from build123d import *

# Parameters (mm, degrees)
F0_W     = 71.2
F0_H     = 88
F1_DEPTH = 1.5
F2_W     = 71.2
F2_H     = 88
F2_W_2   = 67.2
F2_H_2   = 84
F3_DEPTH = 4


with BuildPart() as f1:
    # F0 (on Top) → F1 (new body)
    with BuildSketch(Plane.XY):
        with BuildLine():
            Line((35.4853983939, 37.8176547885), (-32.7146016061, 37.8176547885))
            ThreePointArc((-32.7146016061, 37.8176547885), (-35.5430287309, 36.6460819132), (-36.7146016061, 33.8176547885))
            Line((-36.7146016061, 33.8176547885), (-36.7146016061, -51.1823452115))
            ThreePointArc((-36.7146016061, -51.1823452115), (-35.5430287309, -54.0107723363), (-32.7146016061, -55.1823452115))
            Line((-32.7146016061, -55.1823452115), (35.4853983939, -55.1823452115))
            ThreePointArc((35.4853983939, -55.1823452115), (38.3138255186, -54.0107723363), (39.4853983939, -51.1823452115))
            Line((39.4853983939, -51.1823452115), (39.4853983939, 33.8176547885))
            ThreePointArc((39.4853983939, 33.8176547885), (38.3138255186, 36.6460819132), (35.4853983939, 37.8176547885))
        make_face()
        with Locations((1.3853983939, -8.6823452115)):
            Rectangle(F0_W, F0_H, mode=Mode.SUBTRACT)
        with Locations((1.3853983939, -8.6823452115)):
            Rectangle(F0_W, F0_H)
    extrude(amount=F1_DEPTH)

    # F2 (on face) → F3 (join)
    with BuildSketch(Plane.XY.offset(1.5)):
        with Locations((1.3853983939, -8.6823452115)):
            Rectangle(F2_W, F2_H)
        with Locations((1.3853983939, -8.6823452115)):
            Rectangle(F2_W_2, F2_H_2, mode=Mode.SUBTRACT)
    extrude(amount=F3_DEPTH)


solid = f1.part
The listing builds one solid part. Answer for the finished solid, in the listing's coordinates (mm). A direction names the side the tool comes from. Coordinates: 2 decimals unless noted, no trailing zeros. Order: outer loops, then holes, each group sorted by start corner. A loop starts at its lowest first (then second) coordinate and runs counter-clockwise, first axis right, second up. Notation, with made-up numbers: (34, 45.25) -> (49, 45.25) arc R33 ccw to (49, 77.25) -> close; hole circle Ø8 at (54, -11). An arc over 180 degrees is marked (long way). Answer in a Markdown table with one row per item. Add a question column.
Item 1: Which of the six approach directions +Z, -Z, +X, -X, +Y, -Y give full straight-line access (tool end or side, diameter ignored) to faces 5 (the face through (1, -8, 0)), 6 (the face through (-35.574, -53.98, 0.74)), 7 (the face through (1, -8, 1.5)), 8 (the face through (1, 35.318, 3)), 9 (the face through (-34.215, -9, 3))?
Item 2: Find section C-C (y = -13.5). Write down the section's boundary in (x, z), then the cut area to 3 significant figures.
Item 3: Find section B-B (x = 30.5). Write down the section's boundary in (y, z).
Item 4: Find section A-A (z = 2.35). Write down the section's boundary in (x, y), then the cut area to 3 significant figures.
Item 5: Each of these flat-tipped pins is pushed along its axis until it touches: P1, Ø2, axis at y = -11.5, z = 3.5, coming from the +X side; P2, Ø23, axis at x = 15.5, y = -22.5, coming from the +Z side; P3, Ø1.2, axis at x = 14, z = 4.5, coming from the -Y side. Where does it stop, or does it pass through?
Item 6: Determine the mould class of faces 1 (the face through (36.985, -9, 3)), 2 (the face through (1, -50.682, 3)), 3 (the face through (-35.51, 36.68, 0.74)), 4 (the face through (1, -52.682, 3)) for opening direction Y: +Y half, -Y half, draft (parallel to the pull), parting line (faces both ways), or undercut.
Item 7: Find the intervals of material crossed by L1, parallel to X at y = -42.5, z = 2.2; L2, parallel to Y at x = 32.5, z = 3.65; L3, parallel to Z at x = -6, y = -20, in increasing order. Write a range as from..to.
Result set:
| question | item | result |
|---|---|---|
| 1 | face 5 | -Z, +X, -X, +Y, -Y |
| 1 | face 6 | +Z, -Z, -X, -Y |
| 1 | face 7 | +Z |
| 1 | face 8 | +Z, +X, -X, +Y |
| 1 | face 9 | +Z, -X, +Y, -Y |
| 2 | outline | (-36.71, 0) -> (39.49, 0) -> (39.49, 1.5) -> (36.99, 1.5) -> (36.99, 5.5) -> (34.99, 5.5) -> (34.99, 1.5) -> (-32.21, 1.5) -> (-32.21, 5.5) -> (-34.21, 5.5) -> (-34.21, 1.5) -> (-36.71, 1.5) -> close |
| 2 | area | 130 mm² |
| 3 | outline | (-55.18, 0) -> (37.82, 0) -> (37.82, 1.5) -> (35.32, 1.5) -> (35.32, 5.5) -> (33.32, 5.5) -> (33.32, 1.5) -> (-50.68, 1.5) -> (-50.68, 5.5) -> (-52.68, 5.5) -> (-52.68, 1.5) -> (-55.18, 1.5) -> close |
| 4 | outline | (-34.21, -52.68) -> (36.99, -52.68) -> (36.99, 35.32) -> (-34.21, 35.32) -> close; hole (-32.21, -50.68) -> (34.99, -50.68) -> (34.99, 33.32) -> (-32.21, 33.32) -> close |
| 4 | area | 621 mm² |
| 5 | P1 | stops at x = 36.99 |
| 5 | P2 | stops at z = 1.5 |
| 5 | P3 | stops at y = -52.68 |
| 6 | face 1 | draft |
| 6 | face 2 | undercut |
| 6 | face 3 | +Y half |
| 6 | face 4 | -Y half |
| 7 | L1 | x = -34.21..-32.21, 34.99..36.99 |
| 7 | L2 | y = -52.68..-50.68, 33.32..35.32 |
| 7 | L3 | z = 0..1.5 |
